The model under review builds one solid part; all positions refer to its coordinate system, in mm. A direction names the side the tool comes from. Round coordinates to 2 decimals unless told otherwise and drop trailing zeros. Write each loop counter-clockwise with the first axis right and the second up, starting at its lowest first coordinate (ties: lowest second). Pieces come first, ordered by that corner, then holes. Notation, with made-up numbers: (-13.5, 13) -> (-2.5, 13) arc R15 cw to (-2.5, 17) -> close; hole circle Ø11 at (75.5, 77). An arc over 180 degrees is marked (long way). Use CSV: the item, a comma, the result in double quotes. Start each with the question number.
1) Wall thickness on probe 1 along X at (y, z) = (-3, 25); probe 2 along X at (y, z) = (-10.75, 46); probe 3 along Z at (x, y) = (-20.5, -1): over which ranges is each line inside the solid? List them lowest first. Write a range as [from, to].
2) Take a section at C-C, the plane x = 11. Give the boundary of the cut face in (y, z).
3) Mouldability with a two-part tool opening along Z and no side actions: class faces 4 (the face through (-1, 0, -40)), 5 (the face through (0, -6, -107.558)), 6 (the face through (-5.65, -6, 14)), 7 (the face through (-30.2, -6.1, -11.5)) as released by +Z, released by -Z, zero draft, split by the parting line, or undercut.
4) For pin 1 Ø3 at (x, y) = (8, -3) entering from -Z; pin 2 Ø6 at (y, z) = (-6.5, 14) entering from +X; pin 3 Ø1 at (y, z) = (-8, -73) entering from -X, all flat-tipped, find the tip position at first contact; note any pin that passes through.
5) Take a section at A-A, the plane y = -2.75. Give the boundary of the cut face in (x, z).
6) Machinability: for faces 1 (the face through (4.428, -6, 14)), 2 (the face through (-8, -6, 27.637)), 3 (the face through (4.344, -6.136, 60.494)), which of the approach directions +Z, -Z, +X, -X, +Y, -Y give a long, thin tool a straight path to every point of the face, cutting with its end or side? Answer none if there is none.
7) Take a section at B-B, the plane z = 18.5. Give the boundary of the cut face in (x, y).
from build123d import *

# Parameters (mm, degrees)
F0_W     = 10.077599
F0_H     = 27.637042
F1_DEPTH = 12.446


with BuildPart() as f1:
    # F0 (on Front) → F1 (new body)
    with BuildSketch(Plane.XZ):
        with BuildLine():
            Line((-7.481851, 55.732161), (-10.230287, 27.637042))
            Line((-10.230287, 27.637042), (-5.649562, 27.637042))
            Line((-5.649562, 27.637042), (4.428037, 27.637042))
            Line((4.428037, 27.637042), (9.00876, 27.637042))
            Line((9.00876, 27.637042), (6.260325, 55.426773))
            ThreePointArc((6.260325, 55.426773), (4.298209, 60.557292), (0, 63.977458))
            ThreePointArc((0, 63.977458), (-5.105703, 61.09322), (-7.481851, 55.732161))
        make_face()
        with Locations((-0.610762, 13.818521)):
            Rectangle(F0_W, F0_H)
        with BuildLine():
            Line((4.428037, 0), (-5.649562, 0))
            ThreePointArc((-5.649562, 0), (-30.479653, -11.838325), (-36.914442, -38.58291))
            Line((-36.914442, -38.58291), (35.692916, -38.58291))
            ThreePointArc((35.692916, -38.58291), (29.258127, -11.838325), (4.428037, 0))
        make_face()
        with BuildLine():
            Line((35.692916, -38.58291), (-36.914442, -38.58291))
            ThreePointArc((-36.914442, -38.58291), (-40.497037, -65.894576), (-36.914442, -93.206242))
            ThreePointArc((-36.914442, -93.206242), (-29.192835, -103.766309), (-16.672513, -107.558377))
            Line((-16.672513, -107.558377), (16.980784, -107.558377))
            ThreePointArc((16.980784, -107.558377), (28.203918, -102.816569), (35.692916, -93.206242))
            ThreePointArc((35.692916, -93.206242), (39.7692, -65.894576), (35.692916, -38.58291))
        make_face()
    extrude(amount=F1_DEPTH)


solid = f1.part
Values found:
1,probe 1,"[-5.65, 4.43]"
1,probe 2,"[-8.43, 7.19]"
1,probe 3,"[-107.31, -3.66]"
2,outline,"(-12.45, -107.56) -> (0, -107.56) -> (0, -0.68) -> (-12.45, -0.68) -> close"
3,face 4,"zero draft"
3,face 5,"released by -Z"
3,face 6,"undercut"
3,face 7,"undercut"
4,pin 1,"z = -107.56"
4,pin 2,"x = 4.43"
4,pin 3,"x = -40.29"
5,outline,"(-36.91, -93.21) arc R20.63 ccw to (-16.67, -107.56) -> (16.98, -107.56) arc R24.19 ccw to (35.69, -93.21) arc R93.53 ccw to (35.69, -38.58) arc R31.96 ccw to (4.43, 0) -> (4.43, 27.64) -> (9.01, 27.64) -> (6.26, 55.43) arc R10.42 ccw to (0, 63.98) arc R9.33 ccw to (-7.48, 55.73) -> (-10.23, 27.64) -> (-5.65, 27.64) -> (-5.65, 0) arc R31.96 ccw to (-36.91, -38.58) arc R105.9 ccw to start"
6,face 1,"+X, +Y, -Y"
6,face 2,"-X, +Y, -Y"
6,face 3,"+Z, +X, +Y, -Y"
7,outline,"(-5.65, -12.45) -> (4.43, -12.45) -> (4.43, 0) -> (-5.65, 0) -> close"
